Verification items for the finished model (mm, model axes). Round coordinates to 2 decimals unless told otherwise and drop trailing zeros. Order: outer loops, then holes, each group sorted by start corner. A loop starts at its lowest first (then second) coordinate and runs counter-clockwise, first axis right, second up. Notation, with made-up numbers: M 3,78.5 L 31,78.5 A17 cw 31,92.5 Z; hole C -36,-16 d11. An arc over 180 degrees is marked long. Answer as a JSON object with one key per item and string values. Group by question number.
```python
from build123d import *

# Parameters (mm, degrees)
F0_W     = 10
F0_H     = 10
F1_DEPTH = 30
F2_R     = 2
F3_DEPTH = 46.4
F4_R     = 4
F5_DEPTH = 25
F6_R     = 0.5


with BuildPart() as f1:
    # F0 (on Front) → F1 (new body)
    with BuildSketch(Plane.XZ):
        Rectangle(F0_W, F0_H)
    extrude(amount=F1_DEPTH)

    # F2 (on face) → F3 (cut)
    with BuildSketch(Plane.XZ.offset(30)):
        Circle(F2_R)
    extrude(amount=-F3_DEPTH, mode=Mode.SUBTRACT)

    # F4 (on face) → F5 (cut)
    with BuildSketch(Plane.YZ.offset(5)):
        with Locations((-15, 0)):
            Circle(F4_R)
    extrude(amount=-F5_DEPTH, mode=Mode.SUBTRACT)

    # F6
    f6_edges = [f1.edges().sort_by_distance(p)[0] for p in [
        (-5, -15, 5),
        (5, -15, -5),
        (5, -15, 5),
        (-5, -15, -5),
    ]]
    fillet(f6_edges, radius=F6_R)


solid = f1.part
```
Q1. Cross-section at D-D, the plane z = -3.5. Record the cut outline in (x, y), then the cut area to 3 significant figures.
Q2. Release check for a two-part mould opening along X. For faces 1 (the face through (5, -11, -2)), 2 (the face through (0, -24, -2)), 3 (the face through (2.2, 0, 0.1)) record: released by +X, released by -X, zero draft, split by the parting line, or undercut.
Q3. Cross-section at C-C, the plane x = 0. Record the cut outline in (y, z).
Q4. Thickness scan on line 1 (Y direction, x = -2.5, z = 2); line 2 (Z direction, x = -0.5, y = -15); line 3 (Z direction, x = 0, y = -6.5). Record the ranges inside material, lowest first. Write a range as from..to.
Q5. Gauge pin test, flat end, axial feed: pin 1 Ø3 at (y, z) = (-13.5, 0) entering from +X. Record the tip position at first contact, or that the pin passes through.
Q6. Cross-section at B-B, the plane y = -15. Record the cut outline in (x, z), then the cut area to 3 significant figures.
Q7. Cross-section at A-A, the plane z = 0. Record the cut outline in (x, y), then the cut area to 3 significant figures.
Conclusion:
{
 "1": {"outline": "M -5,-30 L 5,-30 L 5,-16.94 L -5,-16.94 Z; M -5,-13.06 L 5,-13.06 L 5,0 L -5,0 Z", "area": "261 mm2"},
 "2": {"face 1": "released by +X", "face 2": "undercut", "face 3": "zero draft"},
 "3": {"outline": "M -30,-5 L 0,-5 L 0,-2 L -11.54,-2 A4 cw -18.46,-2 L -30,-2 Z; M -30,2 L -18.46,2 A4 cw -11.54,2 L 0,2 L 0,5 L -30,5 Z"},
 "4": {"line 1": "-30..-18.46, -11.54..0", "line 2": "-5..-4, 4..5", "line 3": "-5..-2, 2..5"},
 "5": {"pin 1": "through"},
 "6": {"outline": "M -5,-4.5 A0.5 ccw -4.5,-5 L 4.5,-5 A0.5 ccw 5,-4.5 L 5,-4 L -5,-4 Z; M -5,4 L 5,4 L 5,4.5 A0.5 ccw 4.5,5 L -4.5,5 A0.5 ccw -5,4.5 Z", "area": "19.8 mm2"},
 "7": {"outline": "M -5,-30 L -2,-30 L -2,-19 L -5,-19 Z; M -5,-11 L -2,-11 L -2,0 L -5,0 Z; M 2,-30 L 5,-30 L 5,-19 L 2,-19 Z; M 2,-11 L 5,-11 L 5,0 L 2,0 Z", "area": "132 mm2"}
}
